from build123d import *

# Parameters (mm, degrees)
F0_R     = 150
F0_R_2   = 3
F0_W     = 12
F0_H     = 40
F1_DEPTH = 3


with BuildPart() as f1:
    # F0 (on Top) → F1 (new body, symmetric)
    with BuildSketch(Plane.XY):
        Circle(F0_R)
        with Locations((-120, 0)):
            Circle(F0_R_2, mode=Mode.SUBTRACT)
        with Locations((-48, 0)):
            Rectangle(F0_W, F0_H, mode=Mode.SUBTRACT)
        with Locations((48, 0)):
            Rectangle(F0_W, F0_H, mode=Mode.SUBTRACT)
        with Locations((120, 0)):
            Circle(F0_R_2, mode=Mode.SUBTRACT)
    extrude(amount=F1_DEPTH, both=True)


solid = f1.part
Design review of the part built by this model. Coordinates are the model's own, in mm. Coordinates: 2 decimals unless noted, no trailing zeros. Order: outer loops, then holes, each group sorted by start corner. A loop starts at its lowest first (then second) coordinate and runs counter-clockwise, first axis right, second up. Notation, with made-up numbers: (40.25, -38.5) - (74.25, -38.5) arc R18 ccw to (74.25, -12.5) - close; hole circle Ø8 at (66, 4). An arc over 180 degrees is marked (long way). Put each result on its own line as item: value.
1) Take a section at B-B, the plane x = 62.5. Give the boundary of the cut face in (y, z), and give its area (3 significant figures).
Response values:
outline: (-136.36, -3) - (136.36, -3) - (136.36, 3) - (-136.36, 3) - close
area: 1,640 mm²
2) Wall thickness on L1, parallel to Y at x = 120, z = -0.55; L2, parallel to X at y = 14.5, z = 1.85; L3, parallel to Y at x = 89.5, z = 0: over which ranges is each line inside the solid? List them lowest first. Write a range as from..to.
Response values:
L1: y = -90..-3, 3..90
L2: x = -149.3..-54, -42..42, 54..149.3
L3: y = -120.37..120.37
3) Take a section at A-A, the plane z = 1.55. Give the boundary of the cut face in (x, y).
Response values:
outline: circle Ø300 at (0, 0); hole circle Ø6 at (-120, 0); hole (-54, -20) - (-42, -20) - (-42, 20) - (-54, 20) - close; hole (42, -20) - (54, -20) - (54, 20) - (42, 20) - close; hole circle Ø6 at (120, 0)
4) Insertion check: P1, Ø1.8, axis at y = 1.5, z = 1, coming from the +X side; P2, Ø3, axis at x = 49.5, z = 0, coming from the -Y side; P3, Ø1.5, axis at x = -72.5, z = -1.5, coming from the +Y side; P4, Ø7, axis at x = 120, y = 0, coming from the +Z side. Each pin has a flat end and moves straight along its axis. Give the tip position at first contact, or say it passes through.
Response values:
P1: stops at x = 150
P2: stops at y = -142.11
P3: stops at y = 131.73
P4: stops at z = 3
5) Take a section at C-C, the plane y = -44. Give the boundary of the cut face in (x, z).
Response values:
outline: (-143.4, -3) - (143.4, -3) - (143.4, 3) - (-143.4, 3) - close
